Design review of the part built by this model. Coordinates are the model's own, in mm. Face numbers are marked on the shaded views. Round coordinates to 2 decimals unless told otherwise and drop trailing zeros. Order: outer loops, then holes, each group sorted by start corner. A loop starts at its lowest first (then second) coordinate and runs counter-clockwise, first axis right, second up. Notation, with made-up numbers: M -13,-12 L 44,-12 A33 cw 44,16 Z; hole C 10.5,1 d9. An arc over 180 degrees is marked long. Write each question's results on one line, items separated by ' | '. Start each with the question number.
Item 1: Take a section at C-C, the plane z = 0.65. Write out the cut boundary in (x, y).
Item 2: Clearance check with flat-ended pins moving along their axes: pin 1 (1.4 mm diameter, centred on y = 3.5, z = 3.5, fed in from -X); pin 2 (1.4 mm diameter, centred on y = 4.5, z = 3.5, fed in from +X); pin 3 (2 mm diameter, centred on x = 3, y = 14, fed in from +Z). State where each tip first meets the part, or that it passes through.
Item 3: Take a section at A-A, the plane x = -3. Write out the cut boundary in (y, z).
Item 4: Wall thickness on line 1 (X direction, y = 14, z = 2.9); line 2 (Y direction, x = 5, z = 0.3); line 3 (Y direction, x = -3.5, z = 2.5): over which ranges is each line inside the solid? List them lowest first. Write a range as [from, to].
Item 5: The part is to be moulded in two halves that separate along X. For the marked faces 1, 2, 3 and 4, say which applies: +X half, -X half, draft (parallel to the pull), parting line (faces both ways), or undercut.
Item 6: Take a section at D-D, the plane x = 0.5. Write out the cut boundary in (y, z), plus the area to 3 significant figures.
Item 7: Take a section at B-B, the plane y = -2.5. Write out the cut boundary in (x, z).
```python
from build123d import *
from build123d.topology import SkipClean

# Parameters (mm, degrees)
SKETCH1_R                = 1.25
BOSS_EXTRUDE1_DEPTH      = 4
SKETCH2_R                = 1.65
BOSS_EXTRUDE2_DEPTH      = 3.75
SKETCH2_2_R              = 1.65
CUT_EXTRUDE1_DEPTH       = 19.338824935
MIRROR19_COPY_1_SKETCH_R = 1.25
MIRROR19_COPY_1_DEPTH    = 4
MIRROR19_COPY_2_SKETCH_R = 1.65
MIRROR19_COPY_2_DEPTH    = 3.75
MIRROR19_COPY_3_SKETCH_R = 1.65
MIRROR19_COPY_3_DEPTH    = 19.338824935
MIRROR19_COPY_4_SKETCH_R = 1.65
MIRROR19_COPY_4_DEPTH    = 3.75
MIRROR19_COPY_5_SKETCH_R = 1.65
MIRROR19_COPY_5_DEPTH    = 19.338824935
SKETCH4_W                = 2
SKETCH4_H                = 15.373217597
CUT_EXTRUDE3_DEPTH       = 21.428228019
FILLET1_R                = 1


with BuildPart() as part:
    # Sketch1 → Boss-Extrude1 (new body)
    with BuildSketch(Plane.XY):
        Polygon((0, 0), (-3.75, 0), (-3.75, -10.5), (-6, -10.5), (-6, -17.5), (0, -17.5), align=None)
        with Locations((-3, -14)):
            Circle(SKETCH1_R, mode=Mode.SUBTRACT)
    boss_extrude1 = extrude(amount=BOSS_EXTRUDE1_DEPTH)

    # Sketch2 → Boss-Extrude2 (add, through all)
    with BuildSketch(Plane.ZY.offset(3.75)):
        with Locations((2, -8)):
            Circle(SKETCH2_R)
    boss_extrude2 = extrude(amount=-BOSS_EXTRUDE2_DEPTH)

    # Sketch2<2> → Cut-Extrude1 (cut, through all)
    with BuildSketch(Plane.ZY.offset(3.75)):
        with Locations(Location((2, -8, 0), (0, 0, 270))):
            Circle(SKETCH2_2_R)
    cut_extrude1 = extrude(amount=-CUT_EXTRUDE1_DEPTH, mode=Mode.SUBTRACT)

    # Mirror6: Boss-Extrude1, Boss-Extrude2, Cut-Extrude1 across plane
    add(boss_extrude1.mirror(Plane(origin=(0, -17.5, 4), x_dir=(0, 0, 1), z_dir=(-1, 0, 0))))
    add(boss_extrude2.mirror(Plane(origin=(0, -17.5, 4), x_dir=(0, 0, 1), z_dir=(-1, 0, 0))))
    add(cut_extrude1.mirror(Plane(origin=(0, -17.5, 4), x_dir=(0, 0, 1), z_dir=(-1, 0, 0))), mode=Mode.SUBTRACT)

    # Mirror19: Boss-Extrude1 across plane
    add(boss_extrude1.mirror(Plane.ZX))

    # Mirror19 copy 1 sketch → Mirror19 copy 1 (add)
    with BuildSketch(Plane(origin=(0, 0, 0), x_dir=(-1, 0, 0), z_dir=(0, 0, 1))):
        Polygon((0, 0), (-3.75, 0), (-3.75, -10.5), (-6, -10.5), (-6, -17.5), (0, -17.5), align=None)
        with Locations((-3, -14)):
            Circle(MIRROR19_COPY_1_SKETCH_R, mode=Mode.SUBTRACT)
    extrude(amount=MIRROR19_COPY_1_DEPTH)

    # Mirror19 copy 2 sketch → Mirror19 copy 2 (add, through all)
    with BuildSketch(Plane(origin=(3.75, 0, 0), x_dir=(0, 0, 1), z_dir=(1, 0, 0))):
        with Locations((2, -8)):
            Circle(MIRROR19_COPY_2_SKETCH_R)
    extrude(amount=-MIRROR19_COPY_2_DEPTH)

    # Mirror19 copy 3 sketch → Mirror19 copy 3 (cut, through all)
    with BuildSketch(Plane(origin=(3.75, 0, 0), x_dir=(0, 0, 1), z_dir=(1, 0, 0))):
        with Locations(Location((2, -8, 0), (0, 0, 270))):
            Circle(MIRROR19_COPY_3_SKETCH_R)
    extrude(amount=-MIRROR19_COPY_3_DEPTH, mode=Mode.SUBTRACT)

    # Mirror19 copy 4 sketch → Mirror19 copy 4 (add, through all)
    with BuildSketch(Plane.ZY.offset(3.75)):
        with Locations((2, 8)):
            Circle(MIRROR19_COPY_4_SKETCH_R)
    extrude(amount=-MIRROR19_COPY_4_DEPTH)

    # Mirror19 copy 5 sketch → Mirror19 copy 5 (cut, through all)
    with BuildSketch(Plane.ZY.offset(3.75)):
        with Locations((2, 8)):
            Circle(MIRROR19_COPY_5_SKETCH_R)
    extrude(amount=-MIRROR19_COPY_5_DEPTH, mode=Mode.SUBTRACT)

    # Sketch4 → Cut-Extrude3 (cut, through all)
    with SkipClean():  # the faces are left unmerged after this step: merging them gives an invalid solid
        with BuildSketch(Plane.ZY.offset(3.75)):
            with Locations((2, -0.3266625)):
                Rectangle(SKETCH4_W, SKETCH4_H)
        extrude(amount=-CUT_EXTRUDE3_DEPTH, mode=Mode.SUBTRACT)
    add(part.part.scale(1), mode=Mode.REPLACE)  # the faces are merged on a copy

    # Fillet1
    fillet1_edges = [part.edges().sort_by_distance(p)[0] for p in [
        (-3.75, -10.5, 2),
        (3.75, -10.5, 2),
        (-3.75, 10.5, 2),
        (3.75, 10.5, 2),
    ]]
    fillet(fillet1_edges, radius=FILLET1_R)


solid = part.part
```
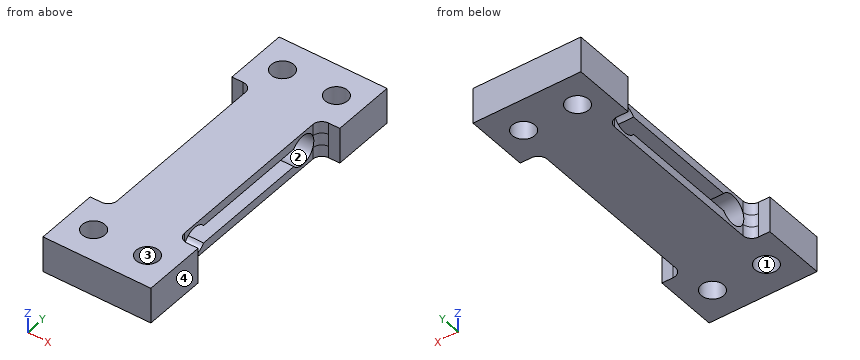
Results list:
1) outline: M -6,-17.5 L 6,-17.5 L 6,-10.5 L 4.75,-10.5 A1 cw 3.75,-9.5 L 3.75,-8.95 L -3.75,-8.95 L -3.75,-9.5 A1 cw -4.75,-10.5 L -6,-10.5 Z; M -6,10.5 L -4.75,10.5 A1 cw -3.75,9.5 L -3.75,8.95 L 3.75,8.95 L 3.75,9.5 A1 cw 4.75,10.5 L 6,10.5 L 6,17.5 L -6,17.5 Z; M -3.75,-7.05 L 3.75,-7.05 L 3.75,7.05 L -3.75,7.05 Z; hole C -3,-14 d2.5; hole C -3,14 d2.5; hole C 3,-14 d2.5; hole C 3,14 d2.5
2) pin 1: x = -3.75 | pin 2: x = 3.75 | pin 3: through
3) outline: M -17.5,0 L -15.25,0 L -15.25,4 L -17.5,4 Z; M -12.75,0 L 12.75,0 L 12.75,4 L -12.75,4 Z; M 15.25,0 L 17.5,0 L 17.5,4 L 15.25,4 Z; hole M -6.69,1 L 6.69,1 A1.65 ccw long 6.69,3 L -6.69,3 A1.65 ccw long Z
4) line 1: [-6, -4.25], [-1.75, 1.75], [4.25, 6] | line 2: [-17.5, -10.5], [10.5, 17.5] | line 3: [-17.5, -15.15], [-12.85, -9.57], [9.57, 12.85], [15.15, 17.5]
5) face 1: undercut | face 2: draft | face 3: undercut | face 4: +X half
6) outline: M -17.5,0 L 17.5,0 L 17.5,4 L -17.5,4 Z; hole M -6.69,1 L 6.69,1 A1.65 ccw long 6.69,3 L -6.69,3 A1.65 ccw long Z | area: 97.1 mm²
7) outline: M -3.75,0 L 3.75,0 L 3.75,1 L -3.75,1 Z; M -3.75,3 L 3.75,3 L 3.75,4 L -3.75,4 Z
